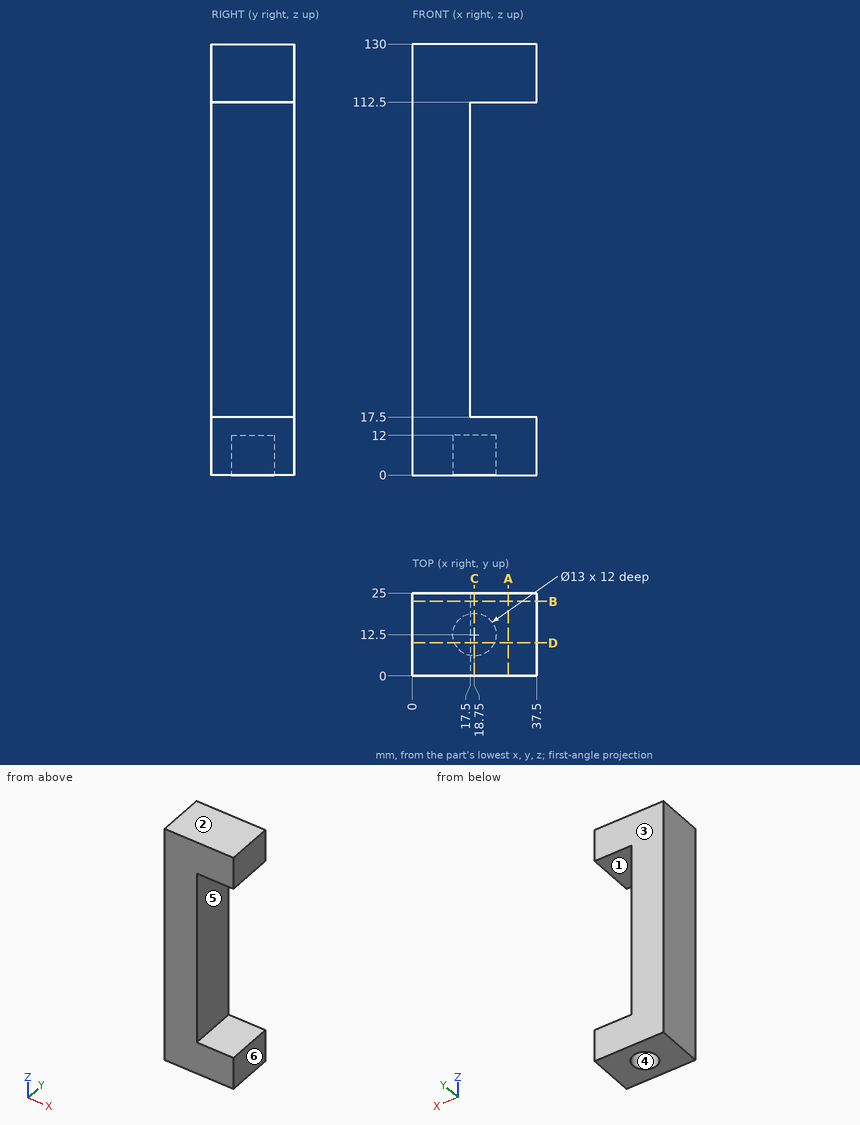
Geometry check sheet. Reference: drawing and pictorial views, mm from the part's lowest x, y, z. A direction names the side the tool comes from. Round coordinates to 2 decimals unless told otherwise and drop trailing zeros. Loops run counter-clockwise (first coordinate to the right, second up) from the corner with the lowest first, then second, coordinate; pieces in that order, holes last. Notation, with made-up numbers: M 78.5,57 L 133.5,57 A19 cw 133.5,93 Z; hole C 32.25,20 d2. An arc over 180 degrees is marked long. Return JSON: item names as keys, results as strings. Group by question number.
(1) Section check A-A, the plane x = 29. Enter the section's corners in (y, z), and give its area (3 significant figures).
(2) Section check D-D, the plane y = 10. Enter the section's corners in (x, z), and give its area (3 significant figures).
(3) Section check B-B, the plane y = 22.5. Enter the section's corners in (x, z), and give its area (4 significant figures).
(4) Mould release check, pull along Z, two halves, no side actions. Record for the marked faces 1, 2 and 3: pulls with the +Z half, pulls with the -Z half, needs draft (parallel to the pull), parting line crosses it, or undercut.
(5) Go/stop test with flat-tipped pins: pin 1 (7.5 mm diameter, centred on y = 16.5, z = 77.5, fed in from +X); pin 2 (6.5 mm diameter, centred on x = 18, y = 9.5, fed in from -Z). Record where each tip stops, or that it passes through.
(6) Scan lines: line 1 along Z through (x, y) = (23, 6); line 2 along Y through (x, z) = (18.75, 3.5); line 3 along X through (y, z) = (12.5, 8.5). Record each from-to range of solid material in increasing order. Write a range as [from, to].
(7) Section check C-C, the plane x = 18.75. Enter the section's corners in (y, z).
(8) Set-up check for the marked faces 4, 5 and 6: record each of +Z, -Z, +X, -X, +Y, -Y from which the full face is reachable in a straight line by a thin tool's end or side.
Data:
{
 "1": {"outline": "M 0,0 L 25,0 L 25,17.5 L 0,17.5 Z; M 0,112.5 L 25,112.5 L 25,130 L 0,130 Z", "area": "875 mm²"},
 "2": {"outline": "M 0,0 L 12.75,0 L 12.75,12 L 24.75,12 L 24.75,0 L 37.5,0 L 37.5,17.5 L 17.5,17.5 L 17.5,112.5 L 37.5,112.5 L 37.5,130 L 0,130 Z", "area": "2,830 mm²"},
 "3": {"outline": "M 0,0 L 37.5,0 L 37.5,17.5 L 17.5,17.5 L 17.5,112.5 L 37.5,112.5 L 37.5,130 L 0,130 Z", "area": "2,975 mm²"},
 "4": {"face 1": "undercut", "face 2": "pulls with the +Z half", "face 3": "needs draft"},
 "5": {"pin 1": "x = 17.5", "pin 2": "z = 12"},
 "6": {"line 1": "[0, 17.5], [112.5, 130]", "line 2": "[0, 6], [19, 25]", "line 3": "[0, 12.25], [25.25, 37.5]"},
 "7": {"outline": "M 0,0 L 6,0 L 6,12 L 19,12 L 19,0 L 25,0 L 25,17.5 L 0,17.5 Z; M 0,112.5 L 25,112.5 L 25,130 L 0,130 Z"},
 "8": {"face 4": "-Z", "face 5": "+X, +Y, -Y", "face 6": "+Z, -Z, +X, +Y, -Y"}
}
